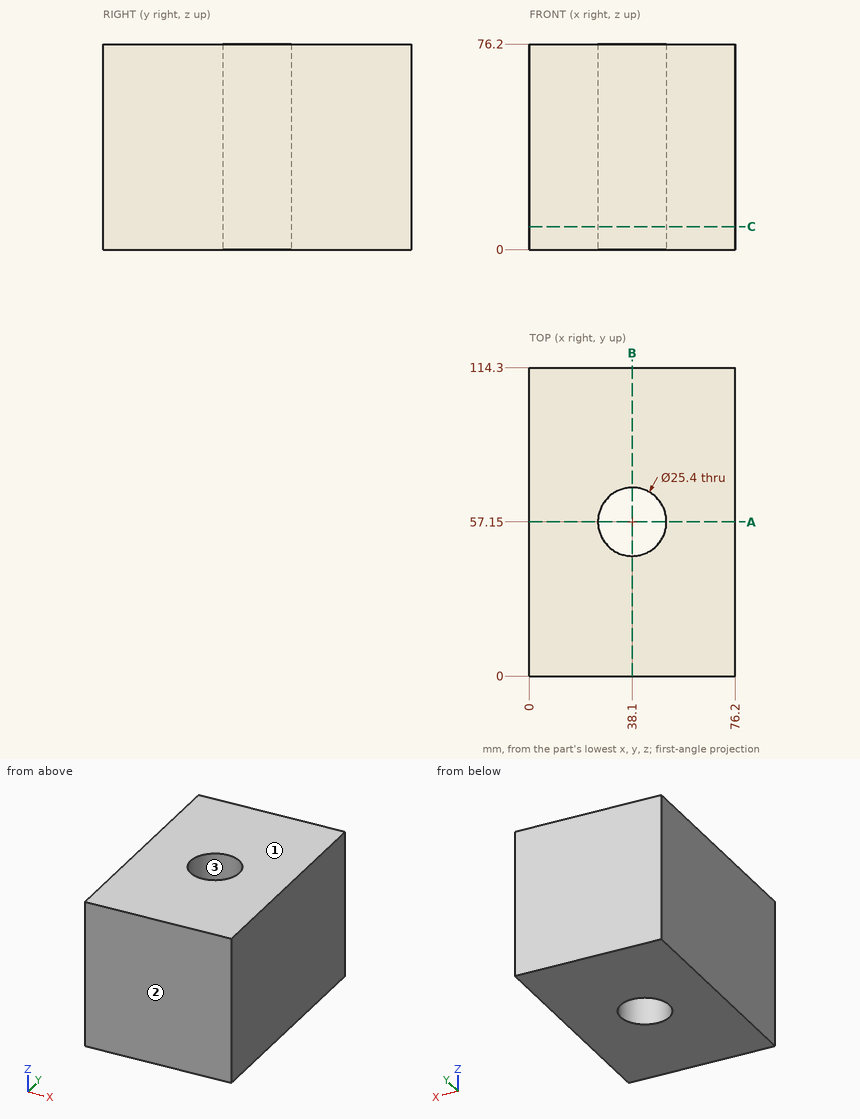
Input: dimensioned drawing with shaded views. Units: mm. Origin: part minimum x, y, z. Coordinates: 2 decimals unless noted, no trailing zeros. Loops run counter-clockwise (first coordinate to the right, second up) from the corner with the lowest first, then second, coordinate; pieces in that order, holes last. Notation, with made-up numbers: (-22.5, 73) -> (25.5, 73) arc R21 cw to (25.5, 107) -> close; hole circle Ø9 at (24, -13.5). An arc over 180 degrees is marked (long way). One line per item, written item: value. Start each with the question number.
Q1. Contact query for a flat-ended pin moving along its axis: P1, Ø3, axis at x = 50, y = 19.5, coming from the -Z side. Output: stop coordinate, or through.
Q2. Line query: line 1 along X through (y, z) = (57.15, 60.5); line 2 along Y through (x, z) = (38, 59); line 3 along Y through (x, z) = (35, 27). Output: solid intervals per line, ascending.
Q3. Section query B-B, the plane x = 38.1. Return the cut outline in (y, z), and give its area (3 significant figures).
Q4. Section query C-C, the plane z = 8.5. Return the cut outline in (x, y).
Q5. Mould query, pull axis Y, two halves, no side actions, for the marked faces 1, 2 and 3. Classes: pulls with the +Y half, pulls with the -Y half, needs draft (parallel to the pull), parting line crosses it, or undercut.
Q6. Section query A-A, the plane y = 57.15. Return the cut outline in (x, z), and give its area (3 significant figures).
Results:
1. P1: z = 0
2. line 1: 0 to 25.4, 50.8 to 76.2
2. line 2: 0 to 44.45, 69.85 to 114.3
2. line 3: 0 to 44.83, 69.47 to 114.3
3. outline: (0, 0) -> (44.45, 0) -> (44.45, 76.2) -> (0, 76.2) -> close; (69.85, 0) -> (114.3, 0) -> (114.3, 76.2) -> (69.85, 76.2) -> close
3. area: 6,770 mm^2
4. outline: (0, 0) -> (76.2, 0) -> (76.2, 114.3) -> (0, 114.3) -> close; hole circle Ø25.4 at (38.1, 57.15)
5. face 1: needs draft
5. face 2: pulls with the -Y half
5. face 3: undercut
6. outline: (0, 0) -> (25.4, 0) -> (25.4, 76.2) -> (0, 76.2) -> close; (50.8, 0) -> (76.2, 0) -> (76.2, 76.2) -> (50.8, 76.2) -> close
6. area: 3,870 mm^2
